Verification items for the finished model (mm, model axes). Face numbers are marked on the shaded views. Give positions to 0.01 mm unless a question says otherwise; leave off trailing zeros. Order: outer loops, then holes, each group sorted by start corner. A loop starts at its lowest first (then second) coordinate and runs counter-clockwise, first axis right, second up.
(1) Scan lines: L1, parallel to X at y = 25, z = -6.25; L2, parallel to Y at x = -25, z = -17.25; L3, parallel to Y at x = -21, z = -2. Record each from-to range of solid material in increasing order.
(2) Gauge pin test, flat ends, axial feed: pin 1 (3.5 mm diameter, centred on x = -25, y = 25, fed in from -Z); pin 2 (2 mm diameter, centred on y = 27, z = -17.5, fed in from +X); pin 3 (1.7 mm diameter, centred on x = -17.5, z = -8, fed in from -Y); pin 4 (1.2 mm diameter, centred on x = -32.5, z = -18, fed in from +Y). Record the tip position at first contact, or that the pin passes through.
(3) Sectioned sample at D-D on z = -20.5. Record the cut outline in (x, y).
(4) Sectioned sample at B-B on z = -2. Record the cut outline in (x, y), plus the area to 3 significant figures.
(5) Mould release check, pull along Y, two halves, no side actions. Record for the marked faces 1, 2 and 3: pulls with the +Y half, pulls with the -Y half, needs draft (parallel to the pull), parting line crosses it, or undercut.
```python
from build123d import *

# Parameters (mm, degrees)
F1_R        = 6.5
F1_R_2      = 5
F2_DEPTH    = 30
F4_W        = 1.5
F4_H        = 2.639524132
F5_DEPTH    = 29.5
F6_COUNT    = 4
F8_R        = 5
F8_R_2      = 2.75
F9_DEPTH    = 1.5
F10_SIZE2   = 1.49999
F10_SIZE    = 9.99999
F10_2_SIZE2 = 1.49999
F10_2_SIZE  = 9.99999
F10_3_SIZE2 = 1.49999
F10_3_SIZE  = 9.99999
F10_4_SIZE2 = 1.49999
F10_4_SIZE  = 9.99999
F11_SIZE    = 0.5
F12_R       = 0.49999


# Not quite as in the source:
# - a fillet or chamfer is up to 0.001 mm smaller than in the source, because OpenCascade refuses the exact size


with BuildPart() as f2:
    # F1 (on offset) → F2 (new body)
    with BuildSketch(Plane.XY):
        with Locations((-25, 25)):
            Circle(F1_R)
        with Locations((-25, 25)):
            Circle(F1_R_2, mode=Mode.SUBTRACT)
    extrude(amount=-F2_DEPTH)

    # F4 (on offset) → F5 (join)
    with BuildSketch(Plane.XY):
        with Locations((-25, 31.680237934)):
            Rectangle(F4_W, F4_H)
    extrude(amount=-F5_DEPTH)

    # F6: F2 ×4 about axis
    f6_axis = Axis((-25, 25, 0), (0, 0, 1))


with BuildPart() as f2_1:
    add(f2.part)
    for i in range(1, F6_COUNT):
        add(f2.part.rotate(f6_axis, i * 360 / F6_COUNT))

    # F8 (on offset) → F9 (join)
    with BuildSketch(Plane.XY.offset(-30)):
        with Locations((-25, 25)):
            Circle(F8_R)
        with Locations((-25, 25)):
            Circle(F8_R_2, mode=Mode.SUBTRACT)
    extrude(amount=F9_DEPTH)

    # F10 (size 10 and 1.5 in the source; OpenCascade refuses exactly that, so slightly less here)
    f10_edges = [f2_1.edges().sort_by_distance(p)[0] for p in [
        (-25, 17, -29.5),
    ]]
    f10_side = f2_1.faces().sort_by_distance((-25, 17, -14.75))[0]
    chamfer(f10_edges, length=F10_SIZE, length2=F10_SIZE2, reference=f10_side)

    # F10#2 (size 10 and 1.5 in the source; OpenCascade refuses exactly that, so slightly less here)
    f10_2_edges = [f2_1.edges().sort_by_distance(p)[0] for p in [
        (-17, 25, -29.5),
    ]]
    f10_2_side = f2_1.faces().sort_by_distance((-17, 25, -14.75))[0]
    chamfer(f10_2_edges, length=F10_2_SIZE, length2=F10_2_SIZE2, reference=f10_2_side)

    # F10#3 (size 10 and 1.5 in the source; OpenCascade refuses exactly that, so slightly less here)
    f10_3_edges = [f2_1.edges().sort_by_distance(p)[0] for p in [
        (-25, 33, -29.5),
    ]]
    f10_3_side = f2_1.faces().sort_by_distance((-25, 33, -14.75))[0]
    chamfer(f10_3_edges, length=F10_3_SIZE, length2=F10_3_SIZE2, reference=f10_3_side)

    # F10#4 (size 10 and 1.5 in the source; OpenCascade refuses exactly that, so slightly less here)
    f10_4_edges = [f2_1.edges().sort_by_distance(p)[0] for p in [
        (-33, 25, -29.5),
    ]]
    f10_4_side = f2_1.faces().sort_by_distance((-33, 25, -14.75))[0]
    chamfer(f10_4_edges, length=F10_4_SIZE, length2=F10_4_SIZE2, reference=f10_4_side)

    # F11
    f11_edges = [f2_1.edges().sort_by_distance(p)[0] for p in [
        (-30, 25, 0),
        (-27.75, 25, -28.5),
    ]]
    chamfer(f11_edges, length=F11_SIZE)

    # F12 (radius 0.5 in the source; OpenCascade refuses exactly that, so slightly less here)
    f12_edges = [f2_1.edges().sort_by_distance(p)[0] for p in [
        (-31.5, 25, -30),
    ]]
    fillet(f12_edges, radius=F12_R)


solid = f2_1.part
```
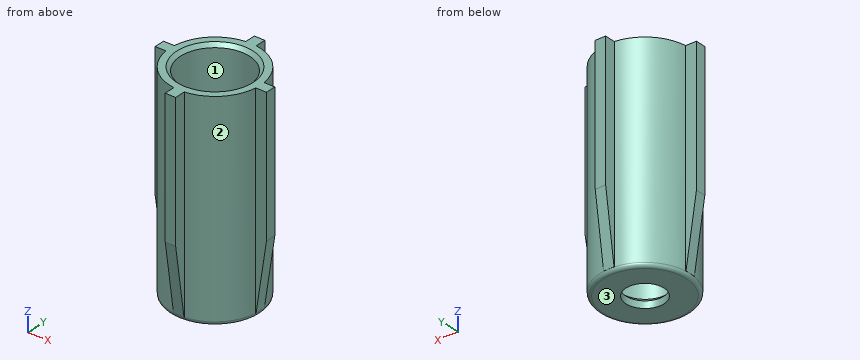
Ans:
1. L1: x = -33 to -30, -20 to -17
1. L2: y = 17 to 20, 30 to 33
1. L3: y = 19.88 to 22, 28 to 30.12
2. pin 1: passes through
2. pin 2: stops at x = -18.58
2. pin 3: stops at y = 24.25
2. pin 4: stops at y = 25.75
3. outline: (-32.85, 24.25) - (-31.46, 24.25) arc R6.5 ccw to (-25.75, 18.54) - (-25.75, 17.15) - (-24.25, 17.15) - (-24.25, 18.54) arc R6.5 ccw to (-18.54, 24.25) - (-17.15, 24.25) - (-17.15, 25.75) - (-18.54, 25.75) arc R6.5 ccw to (-24.25, 31.46) - (-24.25, 32.85) - (-25.75, 32.85) - (-25.75, 31.46) arc R6.5 ccw to (-31.46, 25.75) - (-32.85, 25.75) - close; hole circle Ø10 at (-25, 25)
4. outline: (-33, 24.25) - (-31.46, 24.25) arc R6.5 ccw to (-25.75, 18.54) - (-25.75, 17) - (-24.25, 17) - (-24.25, 18.54) arc R6.5 ccw to (-18.54, 24.25) - (-17, 24.25) - (-17, 25.75) - (-18.54, 25.75) arc R6.5 ccw to (-24.25, 31.46) - (-24.25, 33) - (-25.75, 33) - (-25.75, 31.46) arc R6.5 ccw to (-31.46, 25.75) - (-33, 25.75) - close; hole circle Ø10 at (-25, 25)
4. area: 63.3 mm2
5. face 1: undercut
5. face 2: parting line crosses it
5. face 3: needs draft
